Here's how the part is built. I have some questions about the finished solid (model axes, mm). Give positions to 0.01 mm unless a question says otherwise; leave off trailing zeros. Order: outer loops, then holes, each group sorted by start corner. A loop starts at its lowest first (then second) coordinate and runs counter-clockwise, first axis right, second up. Notation, with made-up numbers: M 56.5,27.25 L 91.5,27.25 A19 ccw 91.5,45.25 Z; hole C -24.5,24 d9. An arc over 180 degrees is marked long. Use one line per item in the form item = value.
from build123d import *

# Parameters (mm, degrees)
SKETCH2_W                        = 250
SKETCH2_H                        = 20
BOSS_EXTRUDE1_DEPTH              = 1000
BOSS_EXTRUDE2_DEPTH              = 20
BOSS_EXTRUDE3_DEPTH              = 20
F_10_0MM_DOWEL_HOLE1_D           = 10
F_10_0MM_DOWEL_HOLE1_CSINK_D     = 10.05
F_10_0MM_DOWEL_HOLE1_CSINK_ANGLE = 90


with BuildPart() as part:
    # Sketch2 → Boss-Extrude1 (new body)
    with BuildSketch(Plane.XY):
        Rectangle(SKETCH2_W, SKETCH2_H)
    extrude(amount=-BOSS_EXTRUDE1_DEPTH)

    # Sketch3 → Boss-Extrude2 (add)
    with BuildSketch(Plane.XY):
        with BuildLine():
            Line((88.6, 10), (88.6, 22))
            ThreePointArc((88.6, 22), (81.1, 29.5), (73.6, 22))
            Line((73.6, 22), (73.6, 10))
            Line((73.6, 10), (88.6, 10))
        make_face()
    boss_extrude2 = extrude(amount=-BOSS_EXTRUDE2_DEPTH)

    # Sketch4 → Boss-Extrude3 (add)
    with BuildSketch(Plane.XY):
        with BuildLine():
            Line((-81.4, 10), (-81.4, 22))
            ThreePointArc((-81.4, 22), (-71.4, 32), (-61.4, 22))
            Line((-61.4, 22), (-61.4, 10))
            Line((-61.4, 10), (-81.4, 10))
        make_face()
    boss_extrude3 = extrude(amount=-BOSS_EXTRUDE3_DEPTH)

    # Ø10.0mm Dowel Hole1 (through all)
    with Locations(Plane.XY):
        with Locations((-71.4, 22), (81.1, 22)):
            f_10_0mm_dowel_hole1 = CounterSinkHole(F_10_0MM_DOWEL_HOLE1_D / 2, F_10_0MM_DOWEL_HOLE1_CSINK_D / 2, counter_sink_angle=F_10_0MM_DOWEL_HOLE1_CSINK_ANGLE)

    # Mirror1: Boss-Extrude2, Boss-Extrude3, Ø10.0mm Dowel Hole1 across plane
    add(boss_extrude2.mirror(Plane.XY.offset(-500)))
    add(boss_extrude3.mirror(Plane.XY.offset(-500)))
    add(f_10_0mm_dowel_hole1.mirror(Plane.XY.offset(-500)), mode=Mode.SUBTRACT)


solid = part.part
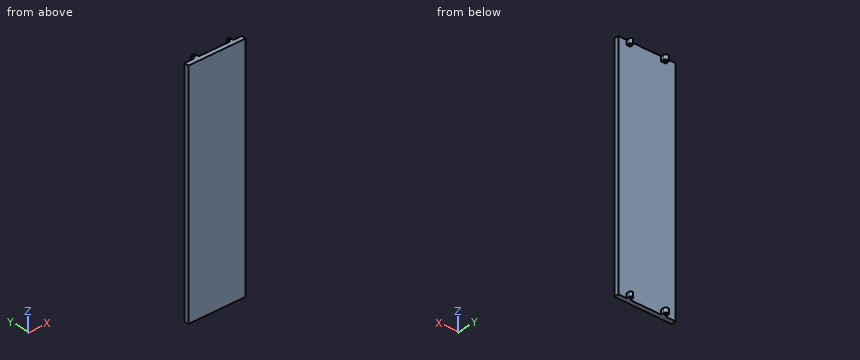
Q1. I'm going to push flat-ended pins straight in: pin 1 Ø3.5 at (y, z) = (16.5, -12.5) entering from -X; pin 2 Ø10 at (x, y) = (-69, 25.5) entering from -Z; pin 3 Ø6 at (y, z) = (18, -6) entering from +X; pin 4 Ø4 at (x, z) = (19, -182.5) entering from +Y. Where does each tip first touch, or does it pass through?
Found:
pin_1 = -81.4
pin_2 = -1000
pin_3 = 88.6
pin_4 = 10
Q2. I want a section at B-B on z = -911. Write out the boundary of the cut face in (x, y).
Found:
outline = M -125,-10 L 125,-10 L 125,10 L -125,10 Z
Q3. I need wall thicknesses on L1, parallel to X at y = 22, z = -9.5; L2, parallel to Y at x = -71.4, z = -10; L3, parallel to Z at x = -75, y = 11. Which ranges of each line are inside material? Lowest first, please.
Found:
L1 = -81.4 to -76.4, -66.4 to -61.4, 73.6 to 76.1, 86.1 to 88.6
L2 = -10 to 17, 27 to 32
L3 = -1000 to -980, -20 to 0
Q4. I want a section at A-A on x = -51. Write out the boundary of the cut face in (y, z), then the cut area to 3 significant figures.
Found:
outline = M -10,-1000 L 10,-1000 L 10,0 L -10,0 Z
area = 20,000 mm²
